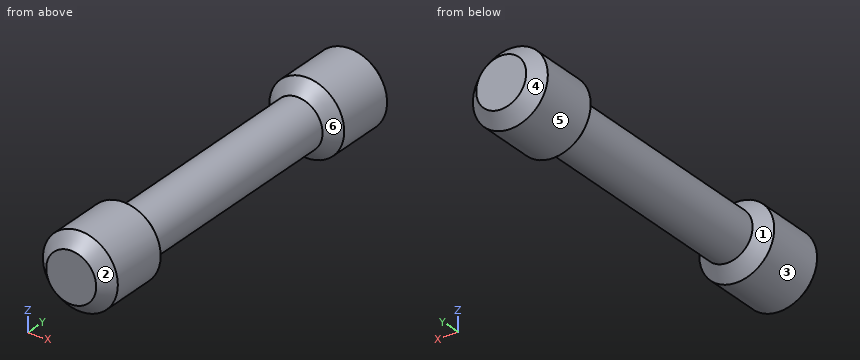
from build123d import *

# Parameters (mm, degrees)
F0_R     = 3
F1_DEPTH = 47
F2_R     = 4.5
F2_R_2   = 3
F3_DEPTH = 10
F4_SIZE  = 1.49999
F5_R     = 4.5
F6_DEPTH = 10
F7_SIZE  = 1.49999


# Not quite as in the source:
# - a fillet or chamfer is up to 0.001 mm smaller than in the source, because OpenCascade refuses the exact size


with BuildPart() as f1:
    # F0 (on Front) → F1 (new body)
    with BuildSketch(Plane.XZ):
        Circle(F0_R)
    extrude(amount=F1_DEPTH)

    # F2 (on face) → F3 (join)
    with BuildSketch(Plane.XZ.offset(47)):
        Circle(F2_R)
        Circle(F2_R_2, mode=Mode.SUBTRACT)
    extrude(amount=-F3_DEPTH)

    # F4 (size 1.5 in the source; OpenCascade refuses exactly that, so slightly less here)
    f4_edges = [f1.edges().sort_by_distance(p)[0] for p in [
        (-4.5, -37, 0),
        (-4.5, -47, 0),
    ]]
    chamfer(f4_edges, length=F4_SIZE)

    # F5 (on face) → F6 (join)
    with BuildSketch(Plane(origin=(0, 0, 0), x_dir=(-1, 0, 0), z_dir=(0, 1, 0))):
        Circle(F5_R)
    extrude(amount=-F6_DEPTH)

    # F7 (size 1.5 in the source; OpenCascade refuses exactly that, so slightly less here)
    f7_edges = [f1.edges().sort_by_distance(p)[0] for p in [
        (4.5, -10, 0),
        (4.5, 0, 0),
    ]]
    chamfer(f7_edges, length=F7_SIZE)


solid = f1.part
Input: part model. Units: mm. Frame: model coordinates. Face numbers are marked on the shaded views. A direction names the side the tool comes from. Give positions to 0.01 mm unless a question says otherwise; leave off trailing zeros. Write each loop counter-clockwise with the first axis right and the second up, starting at its lowest first coordinate (ties: lowest second). Pieces come first, ordered by that corner, then holes.
Q1. Pull-direction query (Y, two-part tool) for the marked faces 1, 2, 3 and 4; classes: pulls with the +Y half, pulls with the -Y half, needs draft (parallel to the pull), parting line crosses it, or undercut.
Q2. Set-up query: the marked faces 5 and 6. Return all of +Z, -Z, +X, -X, +Y, -Y with unobstructed straight access to the full face (end or side cutting, diameter ignored); none if empty.
Q3. Section C-C, the plane y = -41. Output: boundary loops of the cut face in (x, z).
Q4. Material intervals for probe 1 along Y at (x, z) = (-0.5, -3.75); probe 2 along Y at (x, z) = (-1.5, -3.75); probe 3 along Z at (x, y) = (0, -25), sorted ascending.
Q5. First-contact query: P1, Ø1.5, axis at y = -20.5, z = -1, coming from the -X side; P2, Ø1.5, axis at x = -2.5, y = -9, coming from the +Z side; P3, Ø1.5, axis at x = 3.5, y = -19, coming from the +Z side. Flat tips, straight axial feed; report the tip coordinate or a pass-through.
Filled in:
1. face 1: undercut
1. face 2: pulls with the -Y half
1. face 3: needs draft
1. face 4: pulls with the +Y half
2. face 5: +Y, -Y
2. face 6: none
3. outline: circle Ø9 at (0, 0)
4. probe 1: y = -46.22 to -37.78, -9.22 to -0.78
4. probe 2: y = -45.96 to -38.04, -8.96 to -1.04
4. probe 3: z = -3 to 3
5. P1: stops at x = -2.99
5. P2: stops at z = 4.06
5. P3: stops at z = 1.2
